```python
from build123d import *


with BuildPart() as f1:
    # F0 (on Front) → F1 (revolve)
    with BuildSketch(Plane.XZ):
        with BuildLine():
            Line((0, 12), (0, 0))
            Line((0, 0), (23.061637, 0))
            ThreePointArc((23.061637, 0), (28.303251, 1.956368), (30.981233, 6.868629))
            Line((30.981233, 6.868629), (39.83694, 68.858579))
            ThreePointArc((39.83694, 68.858579), (38.988412, 69.989949), (37.857041, 69.141421))
            Line((37.857041, 69.141421), (30.675213, 18.868629))
            ThreePointArc((30.675213, 18.868629), (27.997231, 13.956368), (22.755617, 12))
            Line((22.755617, 12), (0, 12))
        make_face()
    revolve(axis=Axis((0, 0, 45.796357), (0, 0, 1)))


solid = f1.part
```
Model file for the job. Use its own axes, mm. Give positions to 0.01 mm unless a question says otherwise; leave off trailing zeros. Write each loop counter-clockwise with the first axis right and the second up, starting at its lowest first coordinate (ties: lowest second). Pieces come first, ordered by that corner, then holes. Notation, with made-up numbers: (9.5, -29.75) -> (16.5, -29.75) arc R10 cw to (16.5, -12.75) -> close; hole circle Ø6 at (-3.75, 13.25). An arc over 180 degrees is marked (long way). Use CSV: the item, a comma, the result in double quotes. Start each with the question number.
1) Two-plate mould, pull along Y, no slides. Class faces 1 (the flat face through (0, 0, 0)), 2 (the conical face through (32.895, 10.359, 31.41)), 3 (the conical face through (-7.244, -32.623, 38.067)): released by +Y, released by -Y, zero draft, split by the parting line, or undercut.
2) Cut at C-C on z = 27. List the corners of the cut face in (x, y).
3) Pin check, flat tips, straight feed: P1, Ø13.5, axis at x = 0, y = 10, coming from the +Z side; P2, Ø2, axis at y = -23.5, z = 63, coming from the -X side; P3, Ø1, axis at y = 1, z = 61, coming from the -X side. Stop position of each tip, or through.
4) Cut at A-A on x = 0. List the corners of the cut face in (y, z).
5) Cut at D-D on z = 16.5. List the corners of the cut face in (x, y).
6) Drill centre lines: L1, parallel to X at y = -3.5, z = 14.5; L2, parallel to Z at x = 6.5, y = -21; L3, parallel to X at y = -13.5, z = 30. Where is each one in solid material? Low to high.
Final values:
1,face 1,"zero draft"
1,face 2,"split by the parting line"
1,face 3,"undercut"
2,outline,"circle Ø67.71 at (0, 0); hole circle Ø63.67 at (0, 0)"
3,P1,"stops at z = 12"
3,P2,"stops at x = -31.88"
3,P3,"stops at x = -38.77"
4,outline,"(-39.84, 68.86) -> (-30.98, 6.87) arc R8 ccw to (-23.06, 0) -> (23.06, 0) arc R8 ccw to (30.98, 6.87) -> (39.84, 68.86) arc R1 ccw to (37.86, 69.14) -> (30.68, 18.87) arc R8 cw to (22.76, 12) -> (-22.76, 12) arc R8 cw to (-30.68, 18.87) -> (-37.86, 69.14) arc R1 ccw to start"
5,outline,"circle Ø64.71 at (0, 0); hole circle Ø59.9 at (0, 0)"
6,L1,"x = -31.88 to -28.35, 28.35 to 31.88"
6,L2,"z = 0 to 12"
6,L3,"x = -31.52 to -29.31, 29.31 to 31.52"
